Answer from the drawing. Dimensions are ordinates in mm from the lowest x, y and z of the part. A direction names the side the tool comes from. Round coordinates to 2 decimals unless told otherwise and drop trailing zeros. Order: outer loops, then holes, each group sorted by start corner. A loop starts at its lowest first (then second) coordinate and runs counter-clockwise, first axis right, second up. Notation, with made-up numbers: (-5, 40) - (2, 40) arc R16 cw to (2, 67) - close; hole circle Ø2 at (11.25, 4). An arc over 180 degrees is marked (long way). One line per question, with ' | ' between items. Start each with the question number.
1) The part is cut by section D-D, the plane z = 28. Give the vertices of the cut face in (x, y).
2) The part is cut by section C-C, the plane z = 4.5. Give the vertices of the cut face in (x, y).
3) The mould has two halves that part along X. Classify the marked faces 6, 7, 8 and 9: pulls with the +X half, pulls with the -X half, needs draft (parallel to the pull), parting line crosses it, or undercut.
4) For the marked faces 1, 2, 3, 4 and 5, determine the directions among +Z, -Z, +X, -X, +Y, -Y from which every point of the face is accessible in a straight line to the end or side of a thin tool.
5) The part is cut by section A-A, the plane x = 38. Give the vertices of the cut face in (y, z).
6) Flat-ended cylindrical pins translate along their axes: pin 1 (8 mm diameter, centred on x = 93, z = 49.5, fed in from -Y); pin 2 (4.5 mm diameter, centred on y = 45, z = 30, fed in from +X); pin 3 (2 mm diameter, centred on y = 14.5, z = 39.5, fed in from +X); pin 4 (9 mm diameter, centred on y = 40, z = 9.5, fed in from -X). Find the tip coordinate at first contact, or state that the pin passes through.
7) The part is cut by section B-B, the plane y = 44. Give the vertices of the cut face in (x, z), plus the area to 3 significant figures.
8) Straight lines are drawn through the part: line 1 (Y direction, x = 22, z = 31.5); line 2 (X direction, y = 27, z = 11); line 3 (Z direction, x = 39, y = 4). For each, find the intervals that lie inside material, in ascending order. Write a range as from..to.
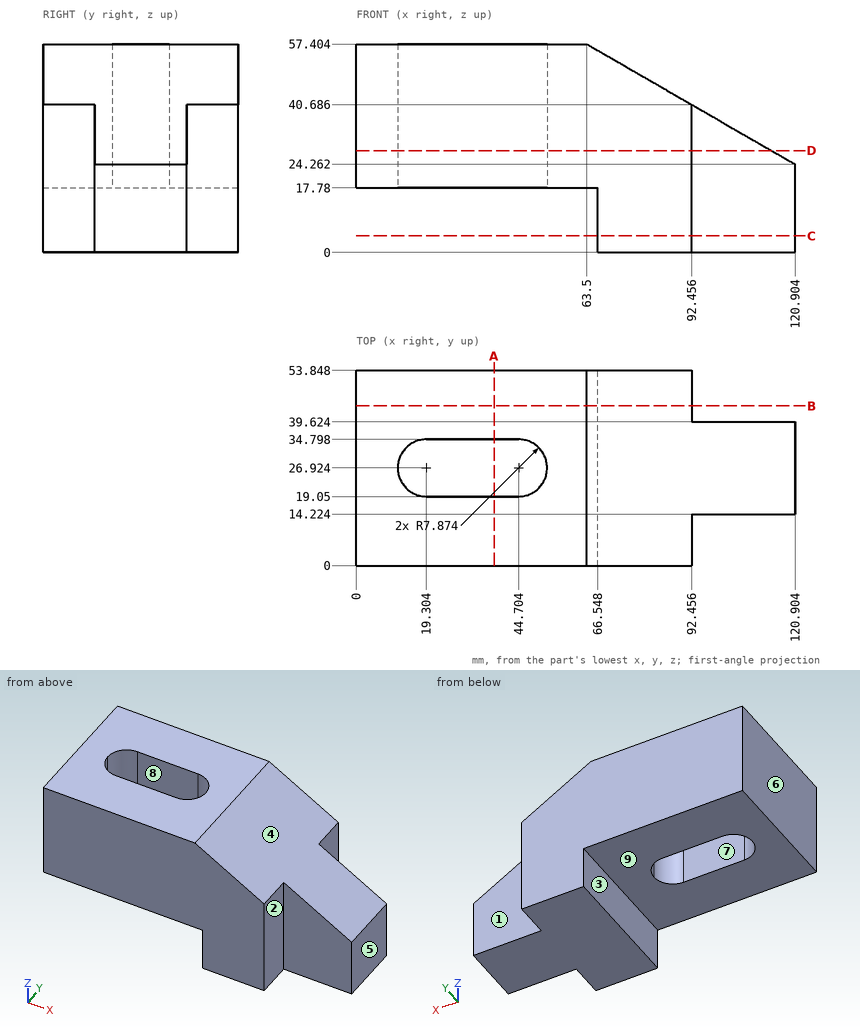
Values:
1) outline: (0, 0) - (92.46, 0) - (92.46, 14.22) - (114.43, 14.22) - (114.43, 39.62) - (92.46, 39.62) - (92.46, 53.85) - (0, 53.85) - close; hole (19.3, 19.05) - (44.7, 19.05) arc R7.87 ccw to (44.7, 34.8) - (19.3, 34.8) arc R7.87 ccw to start
2) outline: (66.55, 0) - (92.46, 0) - (92.46, 14.22) - (120.9, 14.22) - (120.9, 39.62) - (92.46, 39.62) - (92.46, 53.85) - (66.55, 53.85) - close
3) face 6: pulls with the -X half | face 7: undercut | face 8: undercut | face 9: needs draft
4) face 1: +Z, -Z, +X, +Y | face 2: +Z, -Z, +X, -Y | face 3: -Z, -X, +Y, -Y | face 4: +Z, +X, +Y, -Y | face 5: +Z, -Z, +X, +Y, -Y
5) outline: (0, 17.78) - (19.05, 17.78) - (19.05, 57.4) - (0, 57.4) - close; (34.8, 17.78) - (53.85, 17.78) - (53.85, 57.4) - (34.8, 57.4) - close
6) pin 1: passes through | pin 2: stops at x = 92.46 | pin 3: stops at x = 96.24 | pin 4: stops at x = 66.55
7) outline: (0, 17.78) - (66.55, 17.78) - (66.55, 0) - (92.46, 0) - (92.46, 40.69) - (63.5, 57.4) - (0, 57.4) - close | area: 3,880 mm^2
8) line 1: y = 0..19.05, 34.8..53.85 | line 2: x = 66.55..120.9 | line 3: z = 17.78..57.4
